Verification items for the finished model (mm, model axes). Coordinates: 2 decimals unless noted, no trailing zeros. Return JSON: item names as keys, results as strings.
```python
from build123d import *

# Parameters (mm, degrees)
SKETCH1_W             = 400
SKETCH1_H             = 943.901471862
BOSS_EXTRUDE1_DEPTH   = 18
CAVITY1_START         = -439.427247466
CAVITY1_OUTLINE_W     = 50
CAVITY1_OUTLINE_H     = 18
CAVITY1_OUTLINE_W_2   = 200
CAVITY1_DEPTH         = 18
CAVITY1_START_2       = 486.474224396
CAVITY1_2_OUTLINE_W   = 50
CAVITY1_2_OUTLINE_H   = 18
CAVITY1_2_OUTLINE_W_2 = 200
CAVITY1_2_DEPTH       = 18
CAVITY1_START_3       = 7.523488465
CAVITY1_3_OUTLINE_W   = 18
CAVITY1_3_OUTLINE_H   = 18
CAVITY1_3_DEPTH       = 50
CAVITY1_START_4       = -321.427247466
CAVITY1_4_OUTLINE_W   = 18
CAVITY1_4_OUTLINE_H   = 18
CAVITY1_4_DEPTH       = 50
CAVITY1_START_5       = -291.427247466
CAVITY1_5_OUTLINE_W   = 18
CAVITY1_5_OUTLINE_H   = 18
CAVITY1_5_DEPTH       = 50
CAVITY1_START_6       = 306.474224396
CAVITY1_6_OUTLINE_W   = 18
CAVITY1_6_OUTLINE_H   = 18
CAVITY1_6_DEPTH       = 50
CAVITY1_START_7       = 336.474224396
CAVITY1_7_OUTLINE_W   = 18
CAVITY1_7_OUTLINE_H   = 18
CAVITY1_7_DEPTH       = 50
CAVITY1_START_8       = 240.724224396
CAVITY1_8_OUTLINE_W   = 30
CAVITY1_8_OUTLINE_H   = 18
CAVITY1_8_DEPTH       = 18
CAVITY1_START_9       = 270.724224396
CAVITY1_9_OUTLINE_W   = 18
CAVITY1_9_OUTLINE_H   = 18
CAVITY1_9_DEPTH       = 30
CAVITY1_START_10      = 444.474224396
CAVITY1_10_OUTLINE_W  = 18
CAVITY1_10_OUTLINE_H  = 18
CAVITY1_10_DEPTH      = 30
SKETCH3_R             = 3
CUT_EXTRUDE1_DEPTH    = 18
M3_CLEARANCE_HOLE1_D  = 3.4


# Read off the part's stored shape, not the designer's step: Cavity1
with BuildPart() as part:
    # Sketch1 → Boss-Extrude1 (new body)
    with BuildSketch(Plane.XY):
        with Locations((173.181479905, 32.523488465)):
            Rectangle(SKETCH1_W, SKETCH1_H)
    extrude(amount=BOSS_EXTRUDE1_DEPTH)

    # Cavity1 outline → Cavity1 (cut)
    with BuildSketch(Plane(origin=(0, 0, 0), x_dir=(1, 0, 0), z_dir=(0, 1, 0)).offset(CAVITY1_START)):
        with Locations((-1.818520095, -9)):
            Rectangle(CAVITY1_OUTLINE_W, CAVITY1_OUTLINE_H)
        with Locations((173.181479905, -9)):
            Rectangle(CAVITY1_OUTLINE_W_2, CAVITY1_OUTLINE_H)
        with Locations((348.181479905, -9)):
            Rectangle(CAVITY1_OUTLINE_W, CAVITY1_OUTLINE_H)
    extrude(amount=CAVITY1_DEPTH, mode=Mode.SUBTRACT)

    # Cavity1 2 outline → Cavity1 2 (cut)
    with BuildSketch(Plane(origin=(0, 0, 0), x_dir=(1, 0, 0), z_dir=(0, 1, 0)).offset(CAVITY1_START_2)):
        with Locations((-1.818520095, -9)):
            Rectangle(CAVITY1_2_OUTLINE_W, CAVITY1_2_OUTLINE_H)
        with Locations((173.181479905, -9)):
            Rectangle(CAVITY1_2_OUTLINE_W_2, CAVITY1_2_OUTLINE_H)
        with Locations((348.181479905, -9)):
            Rectangle(CAVITY1_2_OUTLINE_W, CAVITY1_2_OUTLINE_H)
    extrude(amount=CAVITY1_2_DEPTH, mode=Mode.SUBTRACT)

    # Cavity1 3 outline → Cavity1 3 (cut)
    with BuildSketch(Plane(origin=(0, 0, 0), x_dir=(1, 0, 0), z_dir=(0, 1, 0)).offset(CAVITY1_START_3)):
        with Locations((202.181479905, -9)):
            Rectangle(CAVITY1_3_OUTLINE_W, CAVITY1_3_OUTLINE_H)
        with Locations((364.181479905, -9)):
            Rectangle(CAVITY1_3_OUTLINE_W, CAVITY1_3_OUTLINE_H)
    extrude(amount=CAVITY1_3_DEPTH, mode=Mode.SUBTRACT)

    # Cavity1 4 outline → Cavity1 4 (cut)
    with BuildSketch(Plane(origin=(0, 0, 0), x_dir=(1, 0, 0), z_dir=(0, 1, 0)).offset(CAVITY1_START_4)):
        with Locations((364.181479905, -9)):
            Rectangle(CAVITY1_4_OUTLINE_W, CAVITY1_4_OUTLINE_H)
    extrude(amount=CAVITY1_4_DEPTH, mode=Mode.SUBTRACT)

    # Cavity1 5 outline → Cavity1 5 (cut)
    with BuildSketch(Plane(origin=(0, 0, 0), x_dir=(1, 0, 0), z_dir=(0, 1, 0)).offset(CAVITY1_START_5)):
        with Locations((202.181479905, -9)):
            Rectangle(CAVITY1_5_OUTLINE_W, CAVITY1_5_OUTLINE_H)
    extrude(amount=CAVITY1_5_DEPTH, mode=Mode.SUBTRACT)

    # Cavity1 6 outline → Cavity1 6 (cut)
    with BuildSketch(Plane(origin=(0, 0, 0), x_dir=(1, 0, 0), z_dir=(0, 1, 0)).offset(CAVITY1_START_6)):
        with Locations((202.181479905, -9)):
            Rectangle(CAVITY1_6_OUTLINE_W, CAVITY1_6_OUTLINE_H)
    extrude(amount=CAVITY1_6_DEPTH, mode=Mode.SUBTRACT)

    # Cavity1 7 outline → Cavity1 7 (cut)
    with BuildSketch(Plane(origin=(0, 0, 0), x_dir=(1, 0, 0), z_dir=(0, 1, 0)).offset(CAVITY1_START_7)):
        with Locations((364.181479905, -9)):
            Rectangle(CAVITY1_7_OUTLINE_W, CAVITY1_7_OUTLINE_H)
    extrude(amount=CAVITY1_7_DEPTH, mode=Mode.SUBTRACT)

    # Cavity1 8 outline → Cavity1 8 (cut)
    with BuildSketch(Plane(origin=(0, 0, 0), x_dir=(1, 0, 0), z_dir=(0, 1, 0)).offset(CAVITY1_START_8)):
        with Locations((67.856479905, -9)):
            Rectangle(CAVITY1_8_OUTLINE_W, CAVITY1_8_OUTLINE_H)
    extrude(amount=CAVITY1_8_DEPTH, mode=Mode.SUBTRACT)

    # Cavity1 9 outline → Cavity1 9 (cut)
    with BuildSketch(Plane(origin=(0, 0, 0), x_dir=(1, 0, 0), z_dir=(0, 1, 0)).offset(CAVITY1_START_9)):
        with Locations((153.531479905, -9)):
            Rectangle(CAVITY1_9_OUTLINE_W, CAVITY1_9_OUTLINE_H)
    extrude(amount=CAVITY1_9_DEPTH, mode=Mode.SUBTRACT)

    # Cavity1 10 outline → Cavity1 10 (cut)
    with BuildSketch(Plane(origin=(0, 0, 0), x_dir=(1, 0, 0), z_dir=(0, 1, 0)).offset(CAVITY1_START_10)):
        with Locations((153.531479905, -9)):
            Rectangle(CAVITY1_10_OUTLINE_W, CAVITY1_10_OUTLINE_H)
    extrude(amount=CAVITY1_10_DEPTH, mode=Mode.SUBTRACT)

    # Sketch3 → Cut-Extrude1 (cut)
    with BuildSketch(Plane.XY.offset(18)):
        with Locations((357.302800248, -273.54856781)):
            Circle(SKETCH3_R)
        with Locations((357.302800248, -319.305927123)):
            Circle(SKETCH3_R)
        with Locations((357.302800248, 384.352904053)):
            Circle(SKETCH3_R)
        with Locations((357.302800248, 338.59554474)):
            Circle(SKETCH3_R)
        with Locations((357.302800248, 55.402168121)):
            Circle(SKETCH3_R)
        with Locations((357.302800248, 9.644808808)):
            Circle(SKETCH3_R)
        with Locations((195.302800248, 354.352904053)):
            Circle(SKETCH3_R)
        with Locations((195.302800248, 308.59554474)):
            Circle(SKETCH3_R)
        with Locations((195.302800248, 55.402168121)):
            Circle(SKETCH3_R)
        with Locations((195.302800248, 9.644808808)):
            Circle(SKETCH3_R)
        with Locations((195.302800248, -243.54856781)):
            Circle(SKETCH3_R)
        with Locations((195.302800248, -289.305927123)):
            Circle(SKETCH3_R)
        with Locations((209.060159561, -289.305927123)):
            Circle(SKETCH3_R)
        with Locations((209.060159561, -243.54856781)):
            Circle(SKETCH3_R)
        with Locations((209.060159561, 9.644808808)):
            Circle(SKETCH3_R)
        with Locations((209.060159561, 55.402168121)):
            Circle(SKETCH3_R)
        with Locations((209.060159561, 308.59554474)):
            Circle(SKETCH3_R)
        with Locations((209.060159561, 354.352904053)):
            Circle(SKETCH3_R)
        with Locations((146.652800248, 472.352904053)):
            Circle(SKETCH3_R)
        with Locations((160.410159561, 472.352904053)):
            Circle(SKETCH3_R)
        with Locations((146.652800248, 446.59554474)):
            Circle(SKETCH3_R)
        with Locations((160.410159561, 446.59554474)):
            Circle(SKETCH3_R)
        with Locations((146.652800248, 298.602904053)):
            Circle(SKETCH3_R)
        with Locations((160.410159561, 298.602904053)):
            Circle(SKETCH3_R)
        with Locations((146.652800248, 272.84554474)):
            Circle(SKETCH3_R)
        with Locations((160.410159561, 272.84554474)):
            Circle(SKETCH3_R)
        with Locations((54.977800248, 256.602904053)):
            Circle(SKETCH3_R)
        with Locations((80.735159561, 256.602904053)):
            Circle(SKETCH3_R)
        with Locations((54.977800248, 242.84554474)):
            Circle(SKETCH3_R)
        with Locations((80.735159561, 242.84554474)):
            Circle(SKETCH3_R)
        with Locations((325.302800248, 488.59554474)):
            Circle(SKETCH3_R)
        with Locations((271.060159561, 488.59554474)):
            Circle(SKETCH3_R)
        with Locations((75.302800248, 488.59554474)):
            Circle(SKETCH3_R)
        with Locations((21.060159561, 488.59554474)):
            Circle(SKETCH3_R)
        with Locations((21.060159561, -423.54856781)):
            Circle(SKETCH3_R)
        with Locations((75.302800248, -423.54856781)):
            Circle(SKETCH3_R)
        with Locations((271.060159561, -423.54856781)):
            Circle(SKETCH3_R)
        with Locations((325.302800248, -423.54856781)):
            Circle(SKETCH3_R)
    extrude(amount=-CUT_EXTRUDE1_DEPTH, mode=Mode.SUBTRACT)

    # M3 Clearance Hole1 (through all)
    with Locations(Plane(origin=(0, 0, 0), x_dir=(-1, 0, 0), z_dir=(0, 0, -1))):
        with Locations((-48.181479905, 495.474224396), (-298.181479905, 495.474224396), (-298.181479905, -430.427247466), (-48.181479905, -430.427247466), (-153.531479905, 372.599224396), (-13.018979905, 249.724224396), (-122.693979905, 249.724224396), (-364.181479905, 436.474224396), (-364.181479905, 196.99885643), (-364.181479905, -131.951879501), (-364.181479905, -371.427247466), (-202.181479905, -371.427247466), (-202.181479905, -116.951879501), (-202.181479905, 181.99885643), (-202.181479905, 436.474224396)):
            Hole(M3_CLEARANCE_HOLE1_D / 2)


solid = part.part
```
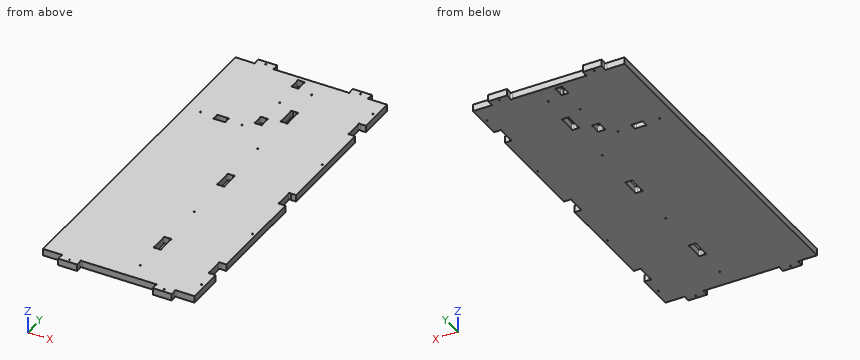
Q1. Cross-section at A-A, the plane z = 4. State how many separate pieces and enclosed holes the cut face has, and give its area (3 significant figures).
Values:
{"separate pieces": "1", "enclosed holes": "21", "area": "359,000 mm^2"}
Q2. Go/stop test with flat-tipped pins: pin 1 (4 mm diameter, centred on x = 368, z = 9.5, fed in from -Y); pin 2 (7 mm diameter, centred on x = 366.5, z = 5, fed in from +Y); pin 3 (1 mm diameter, centred on x = 110, y = 408.5, fed in from -Z). Record where each tip stops, or that it passes through.
Values:
{"pin 1": "y = -421.43", "pin 2": "y = 486.47", "pin 3": "z = 0"}
Q3. Material ranges on line 1 along Y through (x, z) = (298, 10.25); line 2 along X through (y, z) = (-261, 15.75); line 3 along X through (y, z) = (285, 1.5), recorded low to high.
Values:
{"line 1": "-439.43 to -432.12, -428.74 to 493.78, 497.16 to 504.47", "line 2": "-26.82 to 193.18, 211.18 to 373.18", "line 3": "-26.82 to 144.53, 162.53 to 373.18"}
